Autodesk Inventor part; units mm, degrees
ref_plane "Work Plane1" through (0, 160, 0) normal (0, 1, 0) x (1, 0, 0)
ref_plane "YZ Plane" through (0, 0, 0) normal (1, 0, 0) x (0, 1, 0)
ref_plane "XZ Plane" through (0, 0, 0) normal (0, 1, 0) x (-1, 0, 0)
sketch "Sketch1" plane through (0, 0, 0) normal (0, 1, 0) x (-1, 0, 0)
  line L0 (0, 0) -> (-400, 0)
  line L1 (-400, 0) -> (-400, -300)
  line L2 (-400, -300) -> (0, -300)
  line L3 (0, -300) -> (0, 0)
  dimension "d0" = 400
  dimension "d1" = 300
extrude "Extrusion1" add sketch "Sketch1" along normal blind 300
shell "Shell2" thickness 20 removed faces 2 at (0, 100, -200) at (400, 100, -100)
sketch "Sketch2" plane through (0, 0, 0) normal (0, 0, 1) x (1, 0, 0)
  circle A0 centre (50, 15) radius 16.5
  circle A1 centre (350, 15) radius 16.5
  line L0 (0, 0) -> (400, 0)
  dimension "d13" = 33
  dimension "d14" = 33
  dimension "d19" = 15
  dimension "d20" = 15
extrude "Extrusion2" cut sketch "Sketch2" against normal through all
ref_plane "Work Plane1" through (0, 160, 0) normal (0, 1, 0) x (1, 0, 0)
sketch "Sketch3" plane through (0, 160, 0) normal (0, 1, 0) x (1, 0, 0)
  line L0 (400, 300) -> (0, 300)
  line L1 (0, 300) -> (400, 300)
  line L2 (400, 300) -> (400, 0)
  line L3 (400, 0) -> (0, 0)
  line L4 (0, 0) -> (0, 300)
extrude "Extrusion3" add sketch "Sketch3" along normal mid plane 20
Could you check a few things on this model? Use its own coordinates, in mm. A direction names the side the tool comes from. Round coordinates to 2 decimals unless told otherwise and drop trailing zeros. Loops run counter-clockwise (first coordinate to the right, second up) from the corner with the lowest first, then second, coordinate; pieces in that order, holes last.
Q1. I want a section at A-A (y = 176). Write out the boundary of the cut face in (x, z).
Q2. Please list where these lines run through material, in increasing order: L1, parallel to X at y = 15, z = -146; L2, parallel to Y at x = 23.5, z = -93; L3, parallel to Z at x = 104, y = 238.
Q3. I want a section at D-D (x = 242). Write out the boundary of the cut face in (y, z), and give its area (3 significant figures).
Q4. On a 3-axis mill with a long thin cutter (end or side, diameter ignored), from which of +Z, -Z, +X, -X, +Y, -Y can I reach the whole of each face in a straight line? I mean faces 1 (the flat face through (203, 300, -148)), 2 (the flat face through (197, 170, -152)). Say none if no direction works.
Q5. I want a section at B-B (x = 350). Write out the boundary of the cut face in (y, z).
Q6. Thinking about a two-plate mould opening in Z: for faces 3 (the flat face through (383, 20, -148)), 4 (the flat face through (197, 148, 0)), 5 (the flat face through (0, 148, -19)), which applies, pulls with the +Z half, pulls with the -Z half, needs draft (parallel to the pull), parting line crosses it, or undercut?
Q7. I want a section at C-C (z = -209). Write out the boundary of the cut face in (x, y).
Answer below:
1. outline: (0, -300) - (400, -300) - (400, -280) - (0, -280) - close; (0, -20) - (400, -20) - (400, 0) - (0, 0) - close
2. L1: x = 0 to 33.5, 66.5 to 333.5, 366.5 to 400
2. L2: y = 0 to 20, 150 to 170, 280 to 300
2. L3: z = -300 to -280, -20 to 0
3. outline: (0, -300) - (300, -300) - (300, 0) - (0, 0) - close; hole (20, -280) - (150, -280) - (150, -20) - (20, -20) - close; hole (170, -280) - (280, -280) - (280, -20) - (170, -20) - close
3. area: 27,600 mm2
4. face 1: +Z, -Z, +X, -X, +Y
4. face 2: +X, -X
5. outline: (31.5, -300) - (300, -300) - (300, 0) - (31.5, 0) - (31.5, -20) - (150, -20) - (150, -280) - (31.5, -280) - close; hole (170, -280) - (280, -280) - (280, -20) - (170, -20) - close
6. face 3: undercut
6. face 4: pulls with the +Z half
6. face 5: needs draft
7. outline: (0, 0) - (43.13, 0) arc R16.5 cw to (34.28, 20) - (0, 20) - close; (0, 150) - (400, 150) - (400, 170) - (0, 170) - close; (0, 280) - (400, 280) - (400, 300) - (0, 300) - close; (56.87, 0) - (343.13, 0) arc R16.5 cw to (334.28, 20) - (65.72, 20) arc R16.5 cw to start; (356.87, 0) - (400, 0) - (400, 20) - (365.72, 20) arc R16.5 cw to start
